Model file for the job. Use its own axes, mm. Face numbers are marked on the shaded views. A direction names the side the tool comes from. Coordinates: 2 decimals unless noted, no trailing zeros. Order: outer loops, then holes, each group sorted by start corner. A loop starts at its lowest first (then second) coordinate and runs counter-clockwise, first axis right, second up. Notation, with made-up numbers: (-9.75, 59) -> (19.25, 59) arc R25 ccw to (19.25, 84) -> close; hole circle Ø11 at (41.25, -27.5). An arc over 180 degrees is marked (long way). Write item = value, one per line. Start each with the question number.
Q1. 3-axis set-ups, long thin cutter, end or side, ignore diameter. For the marked faces 4 and 5: which of +Z, -Z, +X, -X, +Y, -Y reach the whole face in a straight line?
Q2. Flat gauge pins, fed straight in: pin 1 (10 mm diameter, centred on y = -17, z = 34, fed in from -X); pin 2 (3 mm diameter, centred on y = -11.5, z = -54.5, fed in from -X); pin 3 (3.5 mm diameter, centred on x = 18.5, z = -67.5, fed in from +Y); pin 4 (6.5 mm diameter, centred on y = -10.5, z = -85.6, fed in from +X). Where does each tip first touch, or does it go through?
Q3. Cut at A-A, the plane x = -10. List the corners of the cut face in (y, z).
Q4. Wall check: line 1 (Z direction, x = 19, y = -13.75); line 2 (Z direction, x = -18, y = -10.5); line 3 (Z direction, x = -1.5, y = -15.25). Give the ranges that are in metal, low to high. Write a range as from..to.
Q5. Cut at C-C, the plane z = 21. List the corners of the cut face in (x, y), plus the area to 3 significant figures.
Q6. Cut at D-D, the plane y = -10.5. Give the number of separate pieces and of enclosed holes in the cut face, plus the area to 3 significant figures.
Q7. Mould opens along Z. For the marked faces 1, 2 and 3 say: +Z half, -Z half, draft (parallel to the pull), parting line (faces both ways), or undercut.
Q8. Cut at B-B, the plane y = -18.5. List the corners of the cut face in (x, z).
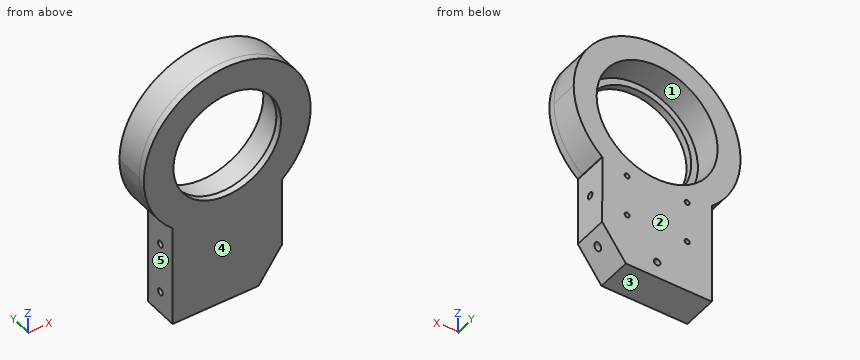
from build123d import *

# Parameters (mm, degrees)
F0_R      = 36.25
F1_DEPTH  = 17
F2_R      = 32.25
F3_DEPTH  = 4
F4_R      = 1.5
F5_DEPTH  = 15
F8_DEPTH  = 25
F11_DEPTH = 25
F13_DEPTH = 12
F15_DEPTH = 25


with BuildPart() as f1:
    # F0 (on Front) → F1 (new body)
    with BuildSketch(Plane.XZ):
        with BuildLine():
            ThreePointArc((33, -37.56328), (45.552168, -20.615528), (50, 0))
            ThreePointArc((50, 0), (0, 50), (-50, 0))
            ThreePointArc((-50, 0), (-45.552168, -20.615528), (-33, -37.56328))
            Line((-33, -37.56328), (-33, -79))
            Line((-33, -79), (-33, -99))
            Line((-33, -99), (-18.995849, -99))
            Line((-18.995849, -99), (0, -99))
            Line((0, -99), (18.995849, -99))
            Line((18.995849, -99), (33, -79))
            Line((33, -79), (33, -37.56328))
        make_face()
        Circle(F0_R, mode=Mode.SUBTRACT)
    extrude(amount=F1_DEPTH)

    # F2 (on face) → F3 (join)
    with BuildSketch(Plane.XZ.offset(17)):
        with BuildLine():
            Line((33, -79), (33, -37.56328))
            ThreePointArc((33, -37.56328), (0, 50), (-33, -37.56328))
            Line((-33, -37.56328), (-33, -99))
            Line((-33, -99), (18.995849, -99))
            Line((18.995849, -99), (33, -79))
        make_face()
        Circle(F2_R, mode=Mode.SUBTRACT)
    extrude(amount=F3_DEPTH)

    # F4 (on face) → F5 (cut)
    with BuildSketch(Plane(origin=(0, 0, 0), x_dir=(-1, 0, 0), z_dir=(0, 1, 0))):
        with Locations((-18, -42.60355)):
            Circle(F4_R)
        with Locations((18, -42.60355)):
            Circle(F4_R)
        with Locations((18, -67.60355)):
            Circle(F4_R)
        with Locations((-18, -67.60355)):
            Circle(F4_R)
    extrude(amount=-F5_DEPTH, mode=Mode.SUBTRACT)

    # F7 (on offset) → F8 (cut)
    with BuildSketch(Plane.YZ.offset(21)):
        with BuildLine():
            ThreePointArc((-12.5, -85.60355), (-10.5, -87.60355), (-8.5, -85.60355))
            Line((-8.5, -85.60355), (-12.5, -85.60355))
        make_face()
        with BuildLine():
            Line((-12.5, -85.60355), (-8.5, -85.60355))
            ThreePointArc((-8.5, -85.60355), (-10.5, -83.60355), (-12.5, -85.60355))
        make_face()
        with BuildLine():
            ThreePointArc((-12.5, -55.10355), (-10.5, -57.10355), (-8.5, -55.10355))
            Line((-8.5, -55.10355), (-12.5, -55.10355))
        make_face()
        with BuildLine():
            Line((-12.5, -55.10355), (-8.5, -55.10355))
            ThreePointArc((-8.5, -55.10355), (-10.5, -53.10355), (-12.5, -55.10355))
        make_face()
    extrude(amount=F8_DEPTH, mode=Mode.SUBTRACT)

    # F10 (on offset) → F11 (cut)
    with BuildSketch(Plane.YZ.offset(-21)):
        with BuildLine():
            ThreePointArc((-12.5, -85.60355), (-10.5, -87.60355), (-8.5, -85.60355))
            Line((-8.5, -85.60355), (-12.5, -85.60355))
        make_face()
        with BuildLine():
            Line((-12.5, -85.60355), (-8.5, -85.60355))
            ThreePointArc((-8.5, -85.60355), (-10.5, -83.60355), (-12.5, -85.60355))
        make_face()
        with BuildLine():
            ThreePointArc((-12.5, -55.10355), (-10.5, -57.10355), (-8.5, -55.10355))
            Line((-8.5, -55.10355), (-12.5, -55.10355))
        make_face()
        with BuildLine():
            Line((-12.5, -55.10355), (-8.5, -55.10355))
            ThreePointArc((-8.5, -55.10355), (-10.5, -53.10355), (-12.5, -55.10355))
        make_face()
    extrude(amount=-F11_DEPTH, mode=Mode.SUBTRACT)

    # F12 (on face) → F13 (cut)
    with BuildSketch(Plane(origin=(0, 0, 0), x_dir=(-1, 0, 0), z_dir=(0, 1, 0))):
        with BuildLine():
            ThreePointArc((0, -87.25), (-2, -89.25), (0, -91.25))
            Line((0, -91.25), (0, -87.25))
        make_face()
        with BuildLine():
            Line((0, -87.25), (0, -91.25))
            ThreePointArc((0, -91.25), (1.414214, -90.664214), (2, -89.25))
            ThreePointArc((2, -89.25), (1.414214, -87.835786), (0, -87.25))
        make_face()
    extrude(amount=-F13_DEPTH, mode=Mode.SUBTRACT)

    # F14 (on face) → F15 (cut)
    with BuildSketch(Plane.XZ.offset(21)):
        Polygon((38.998518, -37.56328), (33, -37.56328), (32.75, -37.56328), (32.948155, -79.000248), (18.745849, -99), (-32.75, -103.90038), (-32.75, -37.56328), (-33, -37.56328), (-37.546977, -48.766561), (-37.546977, -109.624594), (30.626951, -103.313722), (38.998518, -80.774888), align=None)
    extrude(amount=-F15_DEPTH, mode=Mode.SUBTRACT)


solid = f1.part
Here are the results:
q1.face_4 = +Z, -Z, +X, -X, -Y
q1.face_5 = -Z, -X, +Y, -Y
q2.pin_1 = -40.73
q2.pin_2 = -32.75
q2.pin_3 = 0
q2.pin_4 = 30.57
q3.outline = (-21, -99) -> (0, -99) -> (0, -34.84) -> (-17, -34.84) -> (-17, -30.66) -> (-21, -30.66) -> close; (-21, 30.66) -> (-17, 30.66) -> (-17, 34.84) -> (0, 34.84) -> (0, 48.99) -> (-21, 48.99) -> close
q4.line_1 = -98.64..-68.72, -66.49..-43.72, -41.49..-30.87, 30.87..46.25
q4.line_2 = -99..-69.1, -66.1..-44.1, -41.1..-31.47, 31.47..46.65
q4.line_3 = -99..-36.22, 36.22..49.98
q5.outline = (-45.38, -21) -> (-24.48, -21) -> (-24.48, -17) -> (-29.55, -17) -> (-29.55, 0) -> (-45.38, 0) -> close; (24.48, -21) -> (45.38, -21) -> (45.38, 0) -> (29.55, 0) -> (29.55, -17) -> (24.48, -17) -> close
q5.area = 705 mm²
q6.separate_pieces = 1
q6.enclosed_holes = 6
q6.area = 6,840 mm²
q7.face_1 = undercut
q7.face_2 = draft
q7.face_3 = -Z half
q8.outline = (-33, -37.56) -> (-32.75, -37.56) -> (-32.75, -99) -> (18.75, -99) -> (32.95, -79) -> (32.75, -37.56) -> (33, -37.56) arc R50 ccw (long way) to start; hole circle Ø64.5 at (0, 0)
